Autodesk Inventor part; units mm, degrees
ref_plane "Work Plane1" through (0, 11.3, 0) normal (0, 1, 0) x (1, 0, 0)
ref_plane "Work Plane2" through (0, 12.1, 0) normal (0, 1, 0) x (1, 0, 0)
ref_plane "YZ Plane" through (0, 0, 0) normal (1, 0, 0) x (0, 1, 0)
sketch "Sketch1" plane through (0, 0, 0) normal (0, 1, 0) x (-1, 0, 0)
  circle A0 centre (0, 0) radius 1.2
  dimension "d0" = 2.4
extrude "Extrusion1" add sketch "Sketch1" along normal blind 10.6
thread "Thread1"
ref_plane "Work Plane1" through (0, 11.3, 0) normal (0, 1, 0) x (1, 0, 0)
sketch "Sketch3" plane through (0, 11.3, 0) normal (0, 1, 0) x (1, 0, 0)
  circle A0 centre (0, 0) radius 2.15
  dimension "d6" = 4.3
loft "Loft1" add profiles "Sketch3" section 1 edges at (1.2, 10.6, 0)
sketch "Sketch5" plane through (0, 11.3, 0) normal (0, 1, 0) x (1, 0, 0)
  circle A0 centre (0, 0) radius 2.15
extrude "Extrusion2" add sketch "Sketch5" along normal blind 0.7
fillet "Fillet1" radius 2 1 edges at (-2.15, 12, 0)
ref_plane "Work Plane2" through (0, 12.1, 0) normal (0, 1, 0) x (1, 0, 0)
sketch "Sketch7" plane through (0, 12.1, 0) normal (0, 1, 0) x (1, 0, 0)
  line L0 (-1.5, -0.5) -> (-1.5, 0.5)
  line L1 (1.5, 0.5) -> (1.5, -0.5)
  line L2 (-0.5, 1.5) -> (0.5, 1.5)
  line L3 (0.5, -1.5) -> (-0.5, -1.5)
  line L4 (1.5, -0.5) -> (0.5, -0.5)
  line L5 (-0.5, -0.5) -> (-1.5, -0.5)
  line L6 (0.5, 1.5) -> (0.5, 0.5)
  line L7 (0.5, -0.5) -> (0.5, -1.5)
  line L8 (-1.5, 0.5) -> (-0.5, 0.5)
  line L9 (0.5, 0.5) -> (1.5, 0.5)
  line L10 (-0.5, -1.5) -> (-0.5, -0.5)
  line L11 (-0.5, 0.5) -> (-0.5, 1.5)
  dimension "d22" = 3
  dimension "d23" = 1
  dimension "d24" = 3
  dimension "d25" = 1
extrude "Extrusion4" cut sketch "Sketch7" against normal blind 1
equation "\"BendRadius\" = Thickness"
equation "\"BendReliefWidth\" = Thickness"
equation "\"BendReliefDepth\" = 0.5 * Thickness"
equation "\"CornerReliefSize\" = 4 * Thickness"
equation "\"MinimumRemnant\" = 2 * Thickness"
equation "\"TransitionRadius\" = BendRadius"
equation "\"JacobiRadiusSize\" = BendRadius"
equation "\"GapSize\" = Thickness"
properties part number "Parafuso menor Tarraxa"
Source: CAD feature listing. Evaluate the final solid. Frame: model axes, mm. Give positions to 0.01 mm unless a question says otherwise; leave off trailing zeros. Write each loop counter-clockwise with the first axis right and the second up, starting at its lowest first coordinate (ties: lowest second). Pieces come first, ordered by that corner, then holes. Notation, with made-up numbers: M 26,-1.75 L 35,-1.75 A11 ccw 35,4.25 Z; hole C 40,-34 d7. An arc over 180 degrees is marked long. Return JSON: item names as keys, results as strings. Group by question number.
1) Pin query (flat end, axial travel): P1, Ø0.7, axis at y = 11.5, z = 1, coming from the +X side; P2, Ø1.5, axis at x = 0.5, y = 7, coming from the -Z side; P3, Ø0.8, axis at x = 0, y = 11.5, coming from the -Z side; P4, Ø0.7, axis at x = 1, y = 11.5, coming from the +Z side. Return the tip coordinate at first contact, or that it passes through.
2) Cut plane A-A, the plane y = 4.75. Output: boundary loops of the cut face in (x, z).
3) Material intervals for line 1 along X through (y, z) = (1.5, 0); line 2 along Y through (x, z) = (-0.4, -0.15); line 3 along Y through (x, z) = (-1.65, 0.4), sorted ascending. Write a range as [from, to].
4) Pull-direction query (X, two-part tool) for faces 1 (the face through (-0.65, 5.23, -1.01)), 2 (the face through (-1, 11.6, 0.5)), 3 (the face through (0, 0, 0)); classes: pulls with the +X half, pulls with the -X half, needs draft (parallel to the pull), parting line crosses it, or undercut.
Recorded:
{
 "1": {"P1": "stops at x = 2.03", "P2": "stops at z = -1.2", "P3": "stops at z = -2.15", "P4": "stops at z = 2.03"},
 "2": {"outline": "C 0,0 d2.4"},
 "3": {"line 1": "x = [-1.2, 1.2]", "line 2": "y = [0, 11.1]", "line 3": "y = [10.97, 11.69]"},
 "4": {"face 1": "parting line crosses it", "face 2": "undercut", "face 3": "needs draft"}
}
